Verification items for the finished model (mm, model axes). A direction names the side the tool comes from. Round coordinates to 2 decimals unless told otherwise and drop trailing zeros. Loops run counter-clockwise (first coordinate to the right, second up) from the corner with the lowest first, then second, coordinate; pieces in that order, holes last. Notation, with made-up numbers: (-37, 37.5) -> (-20, 37.5) arc R17 cw to (-20, 46.5) -> close; hole circle Ø1 at (-13.75, 87). An arc over 180 degrees is marked (long way). Write item = value, one per line.
```python
from build123d import *

# Parameters (mm, degrees)
F1_DEPTH = 32
F3_DEPTH = 25.4
F5_DEPTH = 25.4


with BuildPart() as f1:
    # F0 (on Front) → F1 (new body)
    with BuildSketch(Plane.XZ):
        Polygon((-10, 21), (-11, 21), (-11, -11), (21, -11), (21, -10), (-10, -10), align=None)
    extrude(amount=F1_DEPTH)

    # F2 (on face) → F3 (cut)
    with BuildSketch(Plane(origin=(-11, 0, 0), x_dir=(0, -1, 0), z_dir=(-1, 0, 0))):
        with BuildLine():
            Line((16, 5), (14.2039487758, 3.2039487758))
            ThreePointArc((14.2039487758, 3.2039487758), (16, 2.46), (17.7960512242, 3.2039487758))
            Line((17.7960512242, 3.2039487758), (16, 5))
        make_face()
        with BuildLine():
            ThreePointArc((14.2039487758, 6.7960512242), (13.46, 5), (14.2039487758, 3.2039487758))
            Line((14.2039487758, 3.2039487758), (16, 5))
            Line((16, 5), (14.2039487758, 6.7960512242))
        make_face()
        with BuildLine():
            Line((14.2039487758, 6.7960512242), (16, 5))
            Line((16, 5), (17.7960512242, 6.7960512242))
            ThreePointArc((17.7960512242, 6.7960512242), (16, 7.54), (14.2039487758, 6.7960512242))
        make_face()
        with BuildLine():
            Line((17.7960512242, 6.7960512242), (16, 5))
            Line((16, 5), (17.7960512242, 3.2039487758))
            ThreePointArc((17.7960512242, 3.2039487758), (18.3466540126, 4.0279840818), (18.54, 5))
            ThreePointArc((18.54, 5), (18.3466540126, 5.9720159182), (17.7960512242, 6.7960512242))
        make_face()
    extrude(amount=-F3_DEPTH, mode=Mode.SUBTRACT)

    # F4 (on face) → F5 (cut)
    with BuildSketch(Plane(origin=(0, 0, -11), x_dir=(1, 0, 0), z_dir=(0, 0, -1))):
        with BuildLine():
            Line((6.7960512242, 17.7960512242), (5, 16))
            Line((5, 16), (6.7960512242, 14.2039487758))
            ThreePointArc((6.7960512242, 14.2039487758), (7.3466540126, 15.0279840818), (7.54, 16))
            ThreePointArc((7.54, 16), (7.3466540126, 16.9720159182), (6.7960512242, 17.7960512242))
        make_face()
        with BuildLine():
            ThreePointArc((6.7960512242, 17.7960512242), (5, 18.54), (3.2039487758, 17.7960512242))
            Line((3.2039487758, 17.7960512242), (5, 16))
            Line((5, 16), (6.7960512242, 17.7960512242))
        make_face()
        with BuildLine():
            Line((6.7960512242, 14.2039487758), (5, 16))
            Line((5, 16), (3.2039487758, 14.2039487758))
            ThreePointArc((3.2039487758, 14.2039487758), (5, 13.46), (6.7960512242, 14.2039487758))
        make_face()
        with BuildLine():
            Line((5, 16), (3.2039487758, 17.7960512242))
            ThreePointArc((3.2039487758, 17.7960512242), (2.46, 16), (3.2039487758, 14.2039487758))
            Line((3.2039487758, 14.2039487758), (5, 16))
        make_face()
    extrude(amount=-F5_DEPTH, mode=Mode.SUBTRACT)


solid = f1.part
```
(1) Sectioned sample at A-A, the plane x = 5. Record the cut outline in (y, z).
Filled sheet:
outline = (-32, -11) -> (-18.54, -11) -> (-18.54, -10) -> (-32, -10) -> close; (-13.46, -11) -> (0, -11) -> (0, -10) -> (-13.46, -10) -> close
(2) Sectioned sample at B-B, the plane y = -28.5. Record the cut outline in (x, z).
Filled sheet:
outline = (-11, -11) -> (21, -11) -> (21, -10) -> (-10, -10) -> (-10, 21) -> (-11, 21) -> close
(3) Material ranges on probe 1 along X at (y, z) = (-6, 6.5), recorded low to high. Write a range as from..to.
Filled sheet:
probe_1 = -11..-10
(4) Sectioned sample at C-C, the plane z = -8. Record the cut outline in (x, y), and give its area (3 significant figures).
Filled sheet:
outline = (-11, -32) -> (-10, -32) -> (-10, 0) -> (-11, 0) -> close
area = 32.0 mm2
(5) Set-up check for faces 1 (the face through (-10, -16, 9)), 2 (the face through (21, -15.8, -10.5)): record each of +Z, -Z, +X, -X, +Y, -Y from which the full face is reachable in a straight line by a thin tool's end or side.
Filled sheet:
face_1 = +Z, +X, +Y, -Y
face_2 = +Z, -Z, +X, +Y, -Y
(6) Go/stop test with flat-tipped pins: pin 1 Ø15.5 at (x, y) = (13, -21) entering from +Z; pin 2 Ø5 at (y, z) = (-21.5, 5) entering from +X. Record where each tip stops, or that it passes through.
Filled sheet:
pin_1 = -10
pin_2 = -10
